CAD build for the part. Positions are in the model's coordinates, mm. Give positions to 0.01 mm unless a question says otherwise; leave off trailing zeros. Loops run counter-clockwise (first coordinate to the right, second up) from the corner with the lowest first, then second, coordinate; pieces in that order, holes last. Notation, with made-up numbers: M 4,-27 L 58,-27 A16 cw 58,-5 Z; hole C 62,-4 d2. An arc over 180 degrees is marked long. Answer as CSV lines item,"result".
from build123d import *

# Parameters (mm, degrees)
SKETCH1_W           = 80
SKETCH1_H           = 80
BOSS_EXTRUDE1_DEPTH = 2.158807247
SKETCH2_W           = 7
SKETCH2_H           = 3.175
CUT_EXTRUDE1_DEPTH  = 3.158807247
CUT_EXTRUDE2_DEPTH  = 3.158807247
SKETCH4_W           = 3.18
SKETCH4_H           = 7
SKETCH4_R           = 1.47
BOSS_EXTRUDE2_DEPTH = 2.158807


with BuildPart() as part:
    # Sketch1 → Boss-Extrude1 (new body)
    with BuildSketch(Plane.XY):
        Rectangle(SKETCH1_W, SKETCH1_H)
    extrude(amount=BOSS_EXTRUDE1_DEPTH)

    # Sketch2 → Cut-Extrude1 (cut, through all)
    with BuildSketch(Plane.XY.offset(2.158807247)):
        with Locations((0, 38.4125)):
            Rectangle(SKETCH2_W, SKETCH2_H)
    extrude(amount=-CUT_EXTRUDE1_DEPTH, mode=Mode.SUBTRACT)

    # Sketch3 → Cut-Extrude2 (cut, through all)
    with BuildSketch(Plane.XY.offset(2.158807247)):
        Polygon((1.47, 34.75), (3.25, 34.75), (3.25, 32.15), (1.47, 32.15), (1.47, 30.075), (-1.47, 30.075), (-1.47, 32.15), (-3.25, 32.15), (-3.25, 34.75), (-1.47, 34.75), (-1.47, 36.825), (1.47, 36.825), align=None)
    extrude(amount=-CUT_EXTRUDE2_DEPTH, mode=Mode.SUBTRACT)

    # Sketch4 → Boss-Extrude2 (add)
    with BuildSketch(Plane.XY.offset(2.158807247)):
        with Locations((-41.59, 0)):
            Rectangle(SKETCH4_W, SKETCH4_H)
        with Locations((-41.59, 0)):
            Circle(SKETCH4_R, mode=Mode.SUBTRACT)
    extrude(amount=-BOSS_EXTRUDE2_DEPTH)


solid = part.part
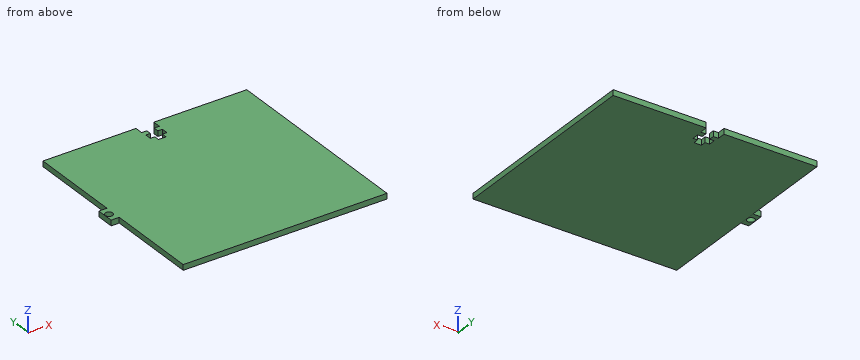
1) Band-saw the part on D-D on y = -27. Give the cut face in (x, z).
Answer below:
outline,"M -40,0 L 40,0 L 40,2.16 L -40,2.16 Z"
2) Band-saw the part on B-B on y = 0. Give the cut face in (x, z), and give its area (3 significant figures).
Answer below:
outline,"M -43.18,0 L -43.06,0 L -43.06,2.16 L -43.18,2.16 Z; M -40.12,0 L 40,0 L 40,2.16 L -40.12,2.16 Z"
area,"173 mm^2"
3) Band-saw the part on A-A on x = -41.59. Give the cut face in (y, z).
Answer below:
outline,"M -3.5,0 L -1.47,0 L -1.47,2.16 L -3.5,2.16 Z; M 1.47,0 L 3.5,0 L 3.5,2.16 L 1.47,2.16 Z"
4) Flat gauge pins, fed straight in: pin 1 (0.9 mm diameter, centred on x = 2, z = 0.5, fed in from +Y) (3 decimals); pin 2 (1 mm diameter, centred on y = 35.5, z = 1.5, fed in from -X). Where does each tip first touch, or does it go through?
Answer below:
pin 1,"stops at y = 36.825"
pin 2,"stops at x = -40"
5) Band-saw the part on C-C on z = 0.4. Give the cut face in (x, y) (3 decimals).
Answer below:
outline,"M -43.18,-3.5 L -40,-3.5 L -40,-40 L 40,-40 L 40,40 L 3.5,40 L 3.5,36.825 L 1.47,36.825 L 1.47,34.75 L 3.25,34.75 L 3.25,32.15 L 1.47,32.15 L 1.47,30.075 L -1.47,30.075 L -1.47,32.15 L -3.25,32.15 L -3.25,34.75 L -1.47,34.75 L -1.47,36.825 L -3.5,36.825 L -3.5,40 L -40,40 L -40,3.5 L -43.18,3.5 Z; hole C -41.59,0 d2.94"
6) Drill centre lines: line 1 (Y direction, x = -41.59, z = 1.15); line 2 (Y direction, x = 2.5, z = 0.4) (3 decimals); line 3 (X direction, y = 26, z = 0.45). Where is each one in solid material? Low to high. Write a range as from..to.
Answer below:
line 1,"y = -3.5..-1.47, 1.47..3.5"
line 2,"y = -40..32.15, 34.75..36.825"
line 3,"x = -40..40"
